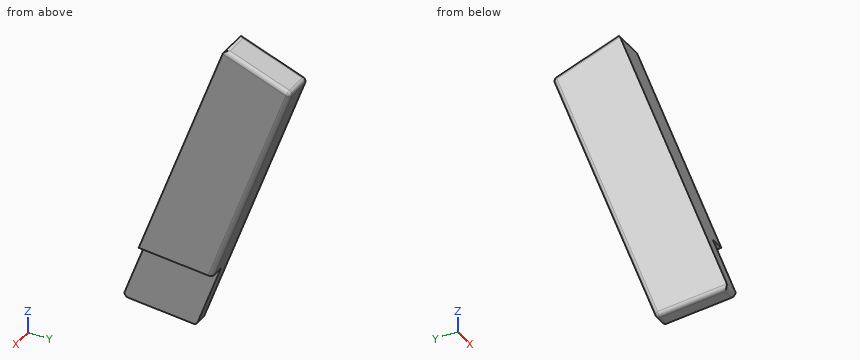
```python
from build123d import *

# Parameters (mm, degrees)
F1_DEPTH = 38.1
F3_DEPTH = 19.05
F4_R     = 5.08


# Not quite as in the source:
# - a feature names something its author has since deleted; it is built from what else it names


with BuildPart() as f1:
    # F0 (on Right) → F1 (new body)
    with BuildSketch(Plane.YZ):
        Polygon((-91.6858274725, 8.0214705098), (0, 0), (128.6780048528, 353.5399127136), (45.1393308649, 383.9455034552), align=None)
    extrude(amount=F1_DEPTH)

    # F2 (on face) → F3 (cut)
    with BuildSketch(Plane.YZ.offset(38.1)):
        Polygon((-92.758420577, 5.074545175), (34.3168153471, -6.0430973832), (0, 0), (30.4055907417, 83.5386739879), (-61.2802367308, 91.5601444977), align=None)
    extrude(amount=-F3_DEPTH, mode=Mode.SUBTRACT)

    # F4
    f4_edges = [f1.edges().sort_by_distance(p)[0] for p in [
        (0, 86.908668, 368.742708),
        (0, 64.339002, 176.769956),
        (38.1, 79.541798, 218.539293),
        (9.525, 0, 0),
        (0, -45.842914, 4.010735),
        (9.525, -91.685827, 8.021471),
        (38.1, 86.908668, 368.742708),
        (19.05, 128.678005, 353.539913),
        (19.05, 45.139331, 383.945503),
    ]]
    fillet(f4_edges, radius=F4_R)


solid = f1.part
```
For this review, take the finished solid that the model builds, in its own axes (mm). Coordinates: 2 decimals unless noted, no trailing zeros. Write each loop counter-clockwise with the first axis right and the second up, starting at its lowest first coordinate (ties: lowest second). Pieces come first, ordered by that corner, then holes. Notation, with made-up numbers: (16.5, 47.25) -> (53.5, 47.25) arc R21 cw to (53.5, 68.25) -> close; hole circle Ø4 at (-27, -26). An arc over 180 degrees is marked (long way). Put each result on its own line as item: value.
Q1. Clearance check with flat-ended pins moving along their axes: pin 1 Ø12 at (x, z) = (5.5, 296) entering from -Y; pin 2 Ø6 at (x, z) = (16.5, 175.5) entering from -Y; pin 3 Ø4 at (x, z) = (16, 104) entering from +Y. State where each tip first meets the part, or that it passes through.
From the geometry:
pin 1: stops at y = 10.95
pin 2: stops at y = -31.82
pin 3: stops at y = 38.58
Q2. Wall thickness on L1, parallel to X at y = -17.5, z = 70.5; L2, parallel to Y at x = 11.5, z = 155.5; L3, parallel to Y at x = 23, z = 353: over which ranges is each line inside the solid? List them lowest first.
From the geometry:
L1: x = 0 to 19.05
L2: y = -38.01 to 56.6
L3: y = 33.88 to 126.59
Q3. Take a section at A-A, the plane x = 13. State the section outline as (y, z) points.
From the geometry:
outline: (-89.42, 14.24) arc R5.08 ccw to (-85.09, 7.44) -> (-3.88, 0.34) arc R5.08 ccw to (1.33, 3.66) -> (126.94, 348.77) arc R5.08 ccw to (123.9, 355.28) -> (49.91, 382.21) arc R5.08 ccw to (43.4, 379.17) -> close
